Autodesk Inventor part; units mm, degrees
ref_plane "YZ Plane" through (0, 0, 0) normal (1, 0, 0) x (0, 1, 0)
ref_plane "XZ Plane" through (0, 0, 0) normal (0, 1, 0) x (-1, 0, 0)
ref_plane "XY Plane" through (0, 0, 0) normal (0, 0, 1) x (1, 0, 0)
ref_plane "Work Plane1" through (500.3579, 35.9816, 443.1665) normal (0, 0, -1) x (0.6678, 0.7444, 0)
sketch "Sketch2" plane through (500.3579, 35.9816, 443.1665) normal (0, 0, -1) x (0.6678, 0.7444, 0)
  line L0 (3.7629, 6.2932) -> (-3.5686, 6.4054)
  line L1 (-3.5686, 6.4054) -> (-7.3315, 0.1122)
  line L2 (-7.3315, 0.1122) -> (-3.7629, -6.2932)
  line L3 (-3.7629, -6.2932) -> (3.5686, -6.4054)
  line L4 (3.5686, -6.4054) -> (7.3315, -0.1122)
  line L5 (7.3315, -0.1122) -> (3.7629, 6.2932)
  line L6 (-7.3315, 0.1122) -> (7.3315, -0.1122)
  line L7 (3.7629, 6.2932) -> (-3.7629, -6.2932)
  line L8 (-3.5686, 6.4054) -> (3.5686, -6.4054)
  line L9 (-3.5686, 6.4054) -> (-5.4229, 9.7337)
  line L10 (-5.4229, 9.7337) -> (5.7182, 9.5632)
  line L11 (5.7182, 9.5632) -> (11.141, -0.1705)
  line L12 (11.141, -0.1705) -> (5.4229, -9.7337)
  line L13 (5.4229, -9.7337) -> (-5.7182, -9.5632)
  line L14 (-5.7182, -9.5632) -> (-11.141, 0.1705)
  line L15 (-11.141, 0.1705) -> (-5.4229, 9.7337)
  point P0 (-360.9105, -348.4198)
  point P1 (0, 0)
  dimension "d0" = 3.81
extrude "Extrusion1" add sketch "Sketch2" against normal blind 7.62
sketch "Sketch3" plane through (500.3579, 35.9816, 443.1665) normal (0, 0, -1) x (-0.7444, 0.6678, 0)
  line L0 (-6.2932, 3.7629) -> (0.1122, 7.3315)
  line L1 (0.1122, 7.3315) -> (6.4054, 3.5686)
  line L2 (6.4054, 3.5686) -> (6.2932, -3.7629)
  line L3 (6.2932, -3.7629) -> (-0.1122, -7.3315)
  line L4 (-0.1122, -7.3315) -> (-6.4054, -3.5686)
  line L5 (-6.4054, -3.5686) -> (-6.2932, 3.7629)
  line L6 (-9.7337, -5.4229) -> (-0.1705, -11.141)
  line L7 (-0.1705, -11.141) -> (9.5632, -5.7182)
  line L8 (9.5632, -5.7182) -> (9.7337, 5.4229)
  line L9 (9.7337, 5.4229) -> (0.1705, 11.141)
  line L10 (0.1705, 11.141) -> (-9.5632, 5.7182)
  line L11 (-9.5632, 5.7182) -> (-9.7337, -5.4229)
  point P0 (348.4198, -360.9105)
sketch "Sketch4" plane through (500.3579, 35.9816, 443.1665) normal (0, 0, -1) x (-0.7444, 0.6678, 0)
  circle A0 centre (0, 0) radius 9.6496
  circle A1 centre (0, 0) radius 3
  point P0 (348.4198, -360.9105)
  dimension "d3" = 6
extrude "Extrusion2" add sketch "Sketch4" along normal blind 0.25
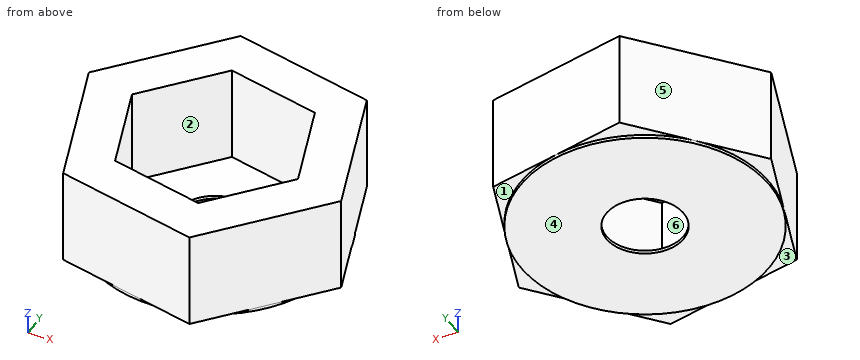
Source: CAD feature listing. Evaluate the final solid. Frame: model axes, mm. Face numbers are marked on the shaded views. A direction names the side the tool comes from. Give positions to 0.01 mm unless a question says otherwise; leave off trailing zeros. Order: outer loops, then holes, each group sorted by start corner. A loop starts at its lowest first (then second) coordinate and runs counter-clockwise, first axis right, second up. Notation, with made-up numbers: (14.5, 86.25) -> (54.5, 86.25) arc R26 ccw to (54.5, 115.25) -> close; hole circle Ø6 at (74.5, 38.5). An arc over 180 degrees is marked (long way). Use a Markdown table: item, result.
Q1. Section C-C (x = 500). Return the cut outline in (y, z).
A:
| item | result |
|---|---|
| outline | (26.22, 443.17) -> (26.34, 443.17) -> (26.34, 442.92) -> (33, 442.92) -> (33, 443.17) -> (29.58, 443.17) -> (29.58, 450.79) -> (26.22, 450.79) -> close; (38.96, 442.92) -> (45.62, 442.92) -> (45.62, 443.17) -> (45.88, 443.17) -> (45.88, 450.79) -> (42.52, 450.79) -> (42.52, 443.17) -> (38.96, 443.17) -> close |
Q2. Material intervals for line 1 (Z direction, x = 495.75, y = 38); line 2 (X direction, y = 36, z = 444); line 3 (Y direction, x = 496.25, z = 447.25), sorted ascending. Write a range as [from, to].
A:
| item | result |
|---|---|
| line 1 | [442.92, 443.17] |
| line 2 | [490.15, 493.64], [507.07, 510.56] |
| line 3 | [26.95, 30.31], [40.93, 45.96] |
Q3. Pull-direction query (X, two-part tool) for the marked faces 4, 5 and 6; classes: +X half, -X half, draft (parallel to the pull), parting line (faces both ways), or undercut.
A:
| item | result |
|---|---|
| face 4 | draft |
| face 5 | -X half |
| face 6 | undercut |
Q4. First-contact query: P1, Ø3, axis at x = 504.5, z = 449, coming from the +Y side; P2, Ø7, axis at x = 500.36, y = 35.98, coming from the +Z side; P3, Ø1.5, axis at x = 498.5, z = 448.5, coming from the +Y side. Flat tips, straight axial feed; report the tip coordinate or a pass-through.
A:
| item | result |
|---|---|
| P1 | y = 45.3 |
| P2 | z = 443.17 |
| P3 | y = 46.32 |
Q5. Access query for the marked faces 1, 2 and 3. Directions: +Z, -Z, +X, -X, +Y, -Y. A direction counts if a zero-diameter tool reaches every point of the face in a straight line with its end or side. Return the directions, or none.
A:
| item | result |
|---|---|
| face 1 | -Z, +X, +Y |
| face 2 | +Z |
| face 3 | -Z, -X, -Y |
Q6. Section A-A (z = 450.25). Return the cut outline in (x, y).
A:
| item | result |
|---|---|
| outline | (489.42, 38.11) -> (493.05, 27.57) -> (503.98, 25.45) -> (511.29, 33.85) -> (507.67, 44.39) -> (496.73, 46.52) -> close; hole (493.16, 37.38) -> (495.55, 30.45) -> (502.74, 29.05) -> (507.56, 34.58) -> (505.17, 41.51) -> (497.97, 42.92) -> close |
Q7. Section B-B (y = 35.5). Return the cut outline in (x, z), and give its area (3 significant figures).
A:
| item | result |
|---|---|
| outline | (490.32, 443.17) -> (490.72, 443.17) -> (490.72, 442.92) -> (497.4, 442.92) -> (497.4, 443.17) -> (493.81, 443.17) -> (493.81, 450.79) -> (490.32, 450.79) -> close; (503.32, 442.92) -> (510, 442.92) -> (510, 443.17) -> (510.73, 443.17) -> (510.73, 450.79) -> (507.24, 450.79) -> (507.24, 443.17) -> (503.32, 443.17) -> close |
| area | 56.5 mm^2 |
Q8. Section D-D (y = 30.75). Return the cut outline in (x, z).
A:
| item | result |
|---|---|
| outline | (491.95, 443.17) -> (492.25, 443.17) -> (492.25, 442.92) -> (508.47, 442.92) -> (508.47, 443.17) -> (508.6, 443.17) -> (508.6, 450.79) -> (504.22, 450.79) -> (504.22, 443.17) -> (495.44, 443.17) -> (495.44, 450.79) -> (491.95, 450.79) -> close |
